Part model, mm, in its own coordinate system. A direction names the side the tool comes from. Coordinates: 2 decimals unless noted, no trailing zeros. Order: outer loops, then holes, each group sorted by start corner. A loop starts at its lowest first (then second) coordinate and runs counter-clockwise, first axis right, second up.
Autodesk Fusion 360 part; units mm, degrees
sketch "Sketch1" plane through (0, 0, 0) normal (1, 0, 0) x (0, 1, 0)
  line L0 (44.3, 0) -> (47.3, 0)
  line L1 (47.3, 0) -> (47.3, 15)
  line L2 (47.3, 15) -> (37.8, 15)
  line L3 (37.8, 15) -> (37.8, 10)
  line L4 (37.8, 10) -> (44.3, 10)
  line L5 (44.3, 10) -> (44.3, 0)
  dimension "d1" = 3
  dimension "d2" = 6.5
  dimension "d3" = 44.3
  dimension "d4" = 10
  dimension "d5" = 5
revolve "Revolve1" add sketch "Sketch1" angle 360 about axis through (0, 0, 1.75) along (0, 0, 1)
sketch "Sketch2" plane through (0, 0, 15) normal (0, 0, 1) x (-1, 0, 0)
  circle A0 centre (0, 0) radius 37.8
  circle A1 centre (0, 0) radius 47.3
  line L0 (46.2308, -10) -> (38.7308, -10)
  line L1 (38.7308, -10) -> (38.7308, 10)
  line L2 (38.7308, 10) -> (46.2308, 10)
  line L3 (46.2308, 10) -> (46.2308, -10)
  line L4 (-38.7308, -10) -> (-46.2308, -10)
  line L5 (-46.2308, -10) -> (-46.2308, 10)
  line L6 (-46.2308, 10) -> (-38.7308, 10)
  line L7 (-38.7308, 10) -> (-38.7308, -10)
  dimension "d7" = 7.5
  dimension "d8" = 20
extrude "Extrude1" add sketch "Sketch2" along normal blind 20 contours L0 L1 L2 L3 | L4 L5 L6 L7
sketch "Sketch3" plane through (46.2308, 0, 0) normal (1, 0, 0) x (0, 1, 0)
  line L0 (-10, 15) -> (10, 15)
  line L1 (10, 15) -> (10, 35)
  line L2 (10, 35) -> (-10, 35)
  line L3 (-10, 35) -> (-10, 15)
  circle A0 centre (0, 25) radius 10
  circle A1 centre (0, 25) radius 3.5
  dimension "d11" = 7
extrude "Extrude2" cut sketch "Sketch3" along normal through all contours L2 L3 A0 | L1 L2 A0 | A1
Q1. Which spindle directions (+Z, -Z, +X, -X, +Y, -Y) get a long thin tool onto all of the face, cutting with end or side? Do faces 1 (the face through (-43.247, -9.603, 4.93)), 2 (the face through (-46.231, 0, 25)), 3 (the face through (-43, 10, 25)), 4 (the face through (43, -10, 25)), 5 (the face through (38.731, 0, 25)). Say none if no direction does.
Results list:
face 1: -Z
face 2: +Z, -X, +Y, -Y
face 3: +Z, +X, -X, +Y
face 4: +Z, +X, -X, -Y
face 5: +Z, +Y, -Y
Q2. Cut at D-D on z = 11.5. Write the cut outline in (x, y), and give its area (3 significant figures).
Results list:
outline: circle Ø94.6 at (0, 0); hole circle Ø75.6 at (0, 0)
area: 2,540 mm2
Q3. Cut at B-B on z = 27.5. Write the cut outline in (x, y).
Results list:
outline: (-46.23, -10) - (-38.73, -10) - (-38.73, 10) - (-46.23, 10) - close; (38.73, -10) - (46.23, -10) - (46.23, 10) - (38.73, 10) - close
Q4. Mould opens along X. For faces 6 (the face through (43, 0, 35)), 7 (the face through (-20, 33, 10)), 8 (the face through (46.231, 0, 25)) say: pulls with the +X half, pulls with the -X half, needs draft (parallel to the pull), parting line crosses it, or undercut.
Results list:
face 6: needs draft
face 7: undercut
face 8: pulls with the +X half
Q5. Cut at A-A on x = 0. Write the cut outline in (y, z), and give its area (3 significant figures).
Results list:
outline: (-47.3, 0) - (-44.3, 0) - (-44.3, 10) - (-37.8, 10) - (-37.8, 15) - (-47.3, 15) - close; (37.8, 10) - (44.3, 10) - (44.3, 0) - (47.3, 0) - (47.3, 15) - (37.8, 15) - close
area: 155 mm2
Q6. Cut at C-C on y = 0. Write the cut outline in (x, z), and give its area (3 significant figures).
Results list:
outline: (-47.3, 0) - (-44.3, 0) - (-44.3, 10) - (-37.8, 10) - (-37.8, 15) - (-38.73, 15) - (-38.73, 35) - (-46.23, 35) - (-46.23, 15) - (-47.3, 15) - close; (37.8, 10) - (44.3, 10) - (44.3, 0) - (47.3, 0) - (47.3, 15) - (46.23, 15) - (46.23, 35) - (38.73, 35) - (38.73, 15) - (37.8, 15) - close
area: 455 mm2
Q7. Wall check: line 1 along X through (y, z) = (0, 11.15); line 2 along X through (y, z) = (0, 4.25). Give the ranges that are in metal, low to high.
Results list:
line 1: x = -47.3 to -37.8, 37.8 to 47.3
line 2: x = -47.3 to -44.3, 44.3 to 47.3
Q8. Pin check, flat tips, straight feed: pin 1 Ø6 at (y, z) = (-3.5, 22.5) entering from +X; pin 2 Ø2 at (x, z) = (-42, 26) entering from -Y; pin 3 Ø6 at (y, z) = (-11.5, 29) entering from -X. Stop position of each tip, or through.
Results list:
pin 1: stops at x = 46.23
pin 2: stops at y = -10
pin 3: stops at x = -46.23
